from build123d import *

# Parameters (mm, degrees)
BOSS_EXTRUDE1_DEPTH              = 50.8
F_6_32_TAPPED_HOLE1_AT_2_COUNT   = 2
F_6_32_TAPPED_HOLE1_AT_2_PITCH   = 40.005
F_6_32_TAPPED_HOLE1_AT_3_COUNT   = 2
F_6_32_TAPPED_HOLE1_AT_3_PITCH   = 179.52019402
F_6_32_TAPPED_HOLE1_AT_4_COUNT   = 2
F_6_32_TAPPED_HOLE1_AT_4_PITCH   = 175.006
BOSS_EXTRUDE2_DEPTH              = 61.976
CUT_EXTRUDE2_DEPTH               = 20.05
F_8_32_TAPPED_HOLE1_AT_2_COUNT   = 2
F_8_32_TAPPED_HOLE1_AT_2_PITCH   = 65.024
F_8_32_TAPPED_HOLE1_AT_3_COUNT   = 2
F_8_32_TAPPED_HOLE1_AT_3_PITCH   = 185.981429482
F_8_32_TAPPED_HOLE1_AT_4_COUNT   = 2
F_8_32_TAPPED_HOLE1_AT_4_PITCH   = 174.244
F_8_32_TAPPED_HOLE1_AT_5_COUNT   = 2
F_8_32_TAPPED_HOLE1_AT_5_PITCH   = 87.122
SKETCH13_W                       = 162.052
SKETCH13_H                       = 63.881
BOSS_EXTRUDE4_DEPTH              = 4.318
F_8_32_TAPPED_HOLE2_AT_2_COUNT   = 2
F_8_32_TAPPED_HOLE2_AT_2_PITCH   = 41.171214069
F_8_32_TAPPED_HOLE2_AT_3_COUNT   = 2
F_8_32_TAPPED_HOLE2_AT_3_PITCH   = 87.455597175
F_8_32_TAPPED_HOLE2_AT_4_COUNT   = 2
F_8_32_TAPPED_HOLE2_AT_4_PITCH   = 81.8388
F_8_32_TAPPED_HOLE2_AT_5_COUNT   = 2
F_8_32_TAPPED_HOLE2_AT_5_PITCH   = 57.868770444
F_8_32_TAPPED_HOLE2_AT_6_COUNT   = 2
F_8_32_TAPPED_HOLE2_AT_6_PITCH   = 41.171214069
CUT_EXTRUDE3_DEPTH               = 3.54
F_1_4_20_TAPPED_HOLE1_AT_2_COUNT = 2
F_1_4_20_TAPPED_HOLE1_AT_2_PITCH = 50.8


with BuildPart() as part:
    # Sketch1 → Boss-Extrude1 (new body)
    with BuildSketch(Plane.XY):
        Polygon((-92.71, 2.54), (92.71, 2.54), (92.71, 0), (110.49, 0), (110.49, 19.05), (92.71, 19.05), (92.71, 74.93), (-92.71, 74.93), (-92.71, 19.05), (-110.49, 19.05), (-110.49, 0), (-92.71, 0), align=None)
    extrude(amount=-BOSS_EXTRUDE1_DEPTH)

    # Sketch3 → #6-32 Tapped Hole1 (revolve, cut)
    with BuildSketch(Plane(origin=(-87.503, 74.93, -45.4025), x_dir=(0, 0, 1), z_dir=(1, 0, 0))):
        Polygon((0, 0), (0, 14.42709403), (1.35255, 13.6144), (1.35255, 9.652), (1.7526, 9.652), (1.7526, 0.635), (2.3876, 0), align=None)
    f_6_32_tapped_hole1 = revolve(axis=Axis((-87.503, 81.28, -45.4025), (0, -1, 0)), mode=Mode.SUBTRACT)

    # #6-32 Tapped Hole1 at 2: #6-32 Tapped Hole1 ×2
    with Locations(*[(0, 0, i * F_6_32_TAPPED_HOLE1_AT_2_PITCH) for i in range(1, F_6_32_TAPPED_HOLE1_AT_2_COUNT)]):
        add(f_6_32_tapped_hole1, mode=Mode.SUBTRACT)

    # #6-32 Tapped Hole1 at 3: #6-32 Tapped Hole1 ×2
    with Locations(*[Vector(0.974854116, 0, 0.22284401) * (i * F_6_32_TAPPED_HOLE1_AT_3_PITCH) for i in range(1, F_6_32_TAPPED_HOLE1_AT_3_COUNT)]):
        add(f_6_32_tapped_hole1, mode=Mode.SUBTRACT)

    # #6-32 Tapped Hole1 at 4: #6-32 Tapped Hole1 ×2
    with Locations(*[(i * F_6_32_TAPPED_HOLE1_AT_4_PITCH, 0, 0) for i in range(1, F_6_32_TAPPED_HOLE1_AT_4_COUNT)]):
        add(f_6_32_tapped_hole1, mode=Mode.SUBTRACT)

    # Sketch5 → Boss-Extrude2 (add)
    with BuildSketch(Plane.XY):
        Polygon((92.71, 74.93), (-92.71, 74.93), (-92.71, 19.05), (-110.49, 19.05), (-110.49, 0), (110.49, 0), (110.49, 19.05), (92.71, 19.05), align=None)
    extrude(amount=BOSS_EXTRUDE2_DEPTH)

    # Sketch16 → Cut-Extrude2 (cut, through all)
    with BuildSketch(Plane(origin=(0, 19.05, 0), x_dir=(1, 0, 0), z_dir=(0, 1, 0))):
        with BuildLine():
            Line((-104.9782, 38.1), (-104.9782, -12.7))
            ThreePointArc((-104.9782, -12.7), (-101.6, -16.0782), (-98.2218, -12.7))
            Line((-98.2218, -12.7), (-98.2218, 38.1))
            ThreePointArc((-98.2218, 38.1), (-101.6, 41.4782), (-104.9782, 38.1))
        make_face()
        with BuildLine():
            Line((104.9782, 38.1), (104.9782, -12.7))
            ThreePointArc((104.9782, -12.7), (101.6, -16.0782), (98.2218, -12.7))
            Line((98.2218, -12.7), (98.2218, 38.1))
            ThreePointArc((98.2218, 38.1), (101.6, 41.4782), (104.9782, 38.1))
        make_face()
    extrude(amount=-CUT_EXTRUDE2_DEPTH, mode=Mode.SUBTRACT)

    # Sketch11 → #8-32 Tapped Hole1 (revolve, cut)
    with BuildSketch(Plane(origin=(-87.122, 69.977, 61.976), x_dir=(0, -1, 0), z_dir=(1, 0, 0))):
        Polygon((0, 0), (0, 17.700206461), (1.7272, 16.6624), (1.7272, 12.7), (2.0828, 12.7), (2.0828, 0.635), (2.7178, 0), align=None)
    f_8_32_tapped_hole1 = revolve(axis=Axis((-87.122, 69.977, 68.326), (0, 0, -1)), mode=Mode.SUBTRACT)

    # #8-32 Tapped Hole1 at 2: #8-32 Tapped Hole1 ×2
    with Locations(*[(0, -i * F_8_32_TAPPED_HOLE1_AT_2_PITCH, 0) for i in range(1, F_8_32_TAPPED_HOLE1_AT_2_COUNT)]):
        add(f_8_32_tapped_hole1, mode=Mode.SUBTRACT)

    # #8-32 Tapped Hole1 at 3: #8-32 Tapped Hole1 ×2
    with Locations(*[Vector(0.936889239, -0.349626305, 0) * (i * F_8_32_TAPPED_HOLE1_AT_3_PITCH) for i in range(1, F_8_32_TAPPED_HOLE1_AT_3_COUNT)]):
        add(f_8_32_tapped_hole1, mode=Mode.SUBTRACT)

    # #8-32 Tapped Hole1 at 4: #8-32 Tapped Hole1 ×2
    with Locations(*[(i * F_8_32_TAPPED_HOLE1_AT_4_PITCH, 0, 0) for i in range(1, F_8_32_TAPPED_HOLE1_AT_4_COUNT)]):
        add(f_8_32_tapped_hole1, mode=Mode.SUBTRACT)

    # #8-32 Tapped Hole1 at 5: #8-32 Tapped Hole1 ×2
    with Locations(*[(i * F_8_32_TAPPED_HOLE1_AT_5_PITCH, 0, 0) for i in range(1, F_8_32_TAPPED_HOLE1_AT_5_COUNT)]):
        add(f_8_32_tapped_hole1, mode=Mode.SUBTRACT)

    # Sketch13 → Boss-Extrude4 (add)
    with BuildSketch(Plane.XY.offset(61.976)):
        with Locations((0, 31.9405)):
            Rectangle(SKETCH13_W, SKETCH13_H)
    extrude(amount=BOSS_EXTRUDE4_DEPTH)

    # Sketch7 → #8-32 Tapped Hole2 (revolve, cut)
    with BuildSketch(Plane(origin=(-40.9194, 52.4002, 66.294), x_dir=(0, -1, 0), z_dir=(1, 0, 0))):
        Polygon((0, 0), (0, 17.700206461), (1.7272, 16.6624), (1.7272, 12.7), (2.0828, 12.7), (2.0828, 0.635), (2.7178, 0), align=None)
    f_8_32_tapped_hole2 = revolve(axis=Axis((-40.9194, 52.4002, 72.644), (0, 0, -1)), mode=Mode.SUBTRACT)

    # #8-32 Tapped Hole2 at 2: #8-32 Tapped Hole2 ×2
    with Locations(*[Vector(0.110431526, -0.993883735, 0) * (i * F_8_32_TAPPED_HOLE2_AT_2_PITCH) for i in range(1, F_8_32_TAPPED_HOLE2_AT_2_COUNT)]):
        add(f_8_32_tapped_hole2, mode=Mode.SUBTRACT)

    # #8-32 Tapped Hole2 at 3: #8-32 Tapped Hole2 ×2
    with Locations(*[Vector(0.883787916, -0.46788772, 0) * (i * F_8_32_TAPPED_HOLE2_AT_3_PITCH) for i in range(1, F_8_32_TAPPED_HOLE2_AT_3_COUNT)]):
        add(f_8_32_tapped_hole2, mode=Mode.SUBTRACT)

    # #8-32 Tapped Hole2 at 4: #8-32 Tapped Hole2 ×2
    with Locations(*[(i * F_8_32_TAPPED_HOLE2_AT_4_PITCH, 0, 0) for i in range(1, F_8_32_TAPPED_HOLE2_AT_4_COUNT)]):
        add(f_8_32_tapped_hole2, mode=Mode.SUBTRACT)

    # #8-32 Tapped Hole2 at 5: #8-32 Tapped Hole2 ×2
    with Locations(*[Vector(0.707106781, -0.707106781, 0) * (i * F_8_32_TAPPED_HOLE2_AT_5_PITCH) for i in range(1, F_8_32_TAPPED_HOLE2_AT_5_COUNT)]):
        add(f_8_32_tapped_hole2, mode=Mode.SUBTRACT)

    # #8-32 Tapped Hole2 at 6: #8-32 Tapped Hole2 ×2
    with Locations(*[Vector(0.993883735, -0.110431526, 0) * (i * F_8_32_TAPPED_HOLE2_AT_6_PITCH) for i in range(1, F_8_32_TAPPED_HOLE2_AT_6_COUNT)]):
        add(f_8_32_tapped_hole2, mode=Mode.SUBTRACT)

    # Sketch17 → Cut-Extrude3 (cut, through all)
    with BuildSketch(Plane.XZ.offset(-2.54)):
        with BuildLine():
            Line((-92.71, 0), (92.71, 0))
            Line((92.71, 0), (92.71, 49.403))
            ThreePointArc((92.71, 49.403), (89.920192091, 56.138192091), (83.185, 58.928))
            Line((83.185, 58.928), (-83.185, 58.928))
            ThreePointArc((-83.185, 58.928), (-89.920192091, 56.138192091), (-92.71, 49.403))
            Line((-92.71, 49.403), (-92.71, 0))
        make_face()
    extrude(amount=CUT_EXTRUDE3_DEPTH, mode=Mode.SUBTRACT)

    # Sketch18 → 1/4-20 Tapped Hole1 (revolve, cut)
    with BuildSketch(Plane(origin=(25.4, 38.1, -50.8), x_dir=(0, 1, 0), z_dir=(1, 0, 0))):
        Polygon((0, 0), (0, 20.583816902), (2.5527, 19.05), (2.5527, 12.7), (3.175, 12.7), (3.175, 0.762), (3.937, 0), align=None)
    f_1_4_20_tapped_hole1 = revolve(axis=Axis((25.4, 38.1, -57.15), (0, 0, 1)), mode=Mode.SUBTRACT)

    # 1/4-20 Tapped Hole1 at 2: 1/4-20 Tapped Hole1 ×2
    with Locations(*[(-i * F_1_4_20_TAPPED_HOLE1_AT_2_PITCH, 0, 0) for i in range(1, F_1_4_20_TAPPED_HOLE1_AT_2_COUNT)]):
        add(f_1_4_20_tapped_hole1, mode=Mode.SUBTRACT)


solid = part.part
Work out the finished part from the listing and answer in its coordinate system (mm). A direction names the side the tool comes from. Round coordinates to 2 decimals unless told otherwise and drop trailing zeros. Write each loop counter-clockwise with the first axis right and the second up, starting at its lowest first coordinate (ties: lowest second). Pieces come first, ordered by that corner, then holes. Notation, with made-up numbers: (-14.75, 18.5) - (36.25, 18.5) arc R27 ccw to (36.25, 37.5) - close; hole circle Ø3 at (-4, 39). An arc over 180 degrees is marked (long way). Answer in a Markdown table with one row per item. Add a question column.
1. A cutting plane is placed at B-B, the plane x = -61. Determine the outline of the cut face in (y, z), and give its area (3 significant figures).
2. A cutting plane is placed at C-C, the plane z = 21. Determine the outline of the cut face in (x, y), and give its area (3 significant figures).
3. Given pin 1 (1 mm diameter, centred on y = 20, z = -5, fed in from +X); pin 2 (4 mm diameter, centred on x = 71, z = -37, fed in from -Y); pin 3 (5.5 mm diameter, centred on x = 87.122, y = 69.977, fed in from +Z); pin 4 (4.5 mm diameter, centred on x = -37.5, y = 10.5, fed in from +Z), each flat-ended and moving along its own axis, determine where each tip first touches the part or whether it passes through.
4. Find the intervals of material crossed by line 1 along X through (y, z) = (38.1, -44.75) (3 decimals); line 2 along Y through (x, z) = (-25.4, -35.5); line 3 along Y through (x, z) = (-56.5, -19), in increasing order. Write a range as from..to.
5. For faces 5 (the flat face through (92.71, 47, 5)), 6 (the cylindrical face through (-89.85, 1.29, 56.21)), 7 (the flat face through (-1, 65, 61.976)), 8 (the flat face through (104.978, 10, -13)), 9 (the flat face through (-89, 5, 49.276)), determine the directions among +Z, -Z, +X, -X, +Y, -Y from which every point of the face is accessible in a straight line to the end or side of a thin tool.
6. The mould has two halves that part along Y. Classify faces 1 (the conical face through (-34, 11, 66)), 2 (the flat face through (-98.222, 10, -12)), 3 (the flat face through (-1, 63.881, 64)), 4 (the cylindrical face through (1.27, 13.13, 59.71)): +Y half, -Y half, draft (parallel to the pull), parting line (faces both ways), or undercut.
7. A cutting plane is placed at A-A, the plane z = -22.5. Determine the outline of the cut face in (x, y), and give its area (3 significant figures).
Worked out:
| question | item | result |
|---|---|---|
| 1 | outline | (0, 58.93) - (2.54, 58.93) - (2.54, -50.8) - (74.93, -50.8) - (74.93, 61.98) - (63.88, 61.98) - (63.88, 66.29) - (0, 66.29) - close |
| 1 | area | 8,450 mm^2 |
| 2 | outline | (-110.49, 0) - (-92.71, 0) - (-92.71, 2.54) - (92.71, 2.54) - (92.71, 0) - (110.49, 0) - (110.49, 19.05) - (92.71, 19.05) - (92.71, 74.93) - (-92.71, 74.93) - (-92.71, 19.05) - (-110.49, 19.05) - close |
| 2 | area | 14,100 mm^2 |
| 3 | pin 1 | x = 92.71 |
| 3 | pin 2 | y = 2.54 |
| 3 | pin 3 | z = 61.98 |
| 3 | pin 4 | z = 66.29 |
| 4 | line 1 | -92.71..-28.575, -22.225..22.225, 28.575..92.71 |
| 4 | line 2 | 2.54..35.55, 40.65..74.93 |
| 4 | line 3 | 2.54..74.93 |
| 5 | face 5 | +Z, -Z, +X, +Y |
| 5 | face 6 | -Z, -Y |
| 5 | face 7 | +Z, +Y |
| 5 | face 8 | +Y, -Y |
| 5 | face 9 | +Z |
| 6 | face 1 | undercut |
| 6 | face 2 | draft |
| 6 | face 3 | +Y half |
| 6 | face 4 | undercut |
| 7 | outline | (-110.49, 0) - (-104.98, 0) - (-104.98, 19.05) - (-110.49, 19.05) - close; (-98.22, 0) - (-92.71, 0) - (-92.71, 2.54) - (92.71, 2.54) - (92.71, 0) - (98.22, 0) - (98.22, 19.05) - (92.71, 19.05) - (92.71, 74.93) - (-92.71, 74.93) - (-92.71, 19.05) - (-98.22, 19.05) - close; (104.98, 0) - (110.49, 0) - (110.49, 19.05) - (104.98, 19.05) - close |
| 7 | area | 13,800 mm^2 |
